Check sheet for the modelled part. Datum: model origin and axes. Units: mm. Face numbers are marked on the shaded views. A direction names the side the tool comes from. Round coordinates to 2 decimals unless told otherwise and drop trailing zeros. Order: outer loops, then holes, each group sorted by start corner. A loop starts at its lowest first (then second) coordinate and runs counter-clockwise, first axis right, second up.
(1) Thickness scan on probe 1 along X at (y, z) = (-25.5, 10); probe 2 along Y at (x, z) = (0, 3.75); probe 3 along X at (y, z) = (-20, 9.75). Record the ranges inside material, lowest first.
(2) Sectioned sample at D-D, the plane x = 42.9. Enter the section's corners in (y, z), and give its area (3 significant figures).
(3) Depth check by flat-ended pin: pin 1 (5 mm diameter, centred on x = 39, z = 5.5, fed in from +Y); pin 2 (5 mm diameter, centred on y = 0.5, z = 2, fed in from -X); pin 3 (5 mm diameter, centred on y = 19, z = 13.5, fed in from -X). Enter the tip coordinate at first touch or a pass-through.
(4) Sectioned sample at B-B, the plane y = -19. Enter the section's corners in (x, z), and give its area (3 significant figures).
(5) Tool access check on the marked faces 1, 2, 3 and 4. Record the directions out of +Z, -Z, +X, -X, +Y, -Y that give a thin tool (end or side, any length) a straight path to the whole face; none if there is none.
(6) Sectioned sample at C-C, the plane z = 5.5. Enter the section's corners in (x, y).
(7) Mould release check, pull along Y, two halves, no side actions. Record for the marked faces 5, 6 and 7: released by +Y, released by -Y, zero draft, split by the parting line, or undercut.
(8) Sectioned sample at A-A, the plane x = -12. Enter the section's corners in (y, z).
```python
from build123d import *
from build123d.topology import SkipClean

# Parameters (mm, degrees)
SKETCH1_W           = 50
SKETCH1_H           = 60
BOSS_EXTRUDE1_DEPTH = 12
SKETCH2_W           = 41
SKETCH2_H           = 4.2
CUT_EXTRUDE1_DEPTH  = 67.098411479
SKETCH3_W           = 12
SKETCH3_H           = 30
BOSS_EXTRUDE2_DEPTH = 42
SKETCH4_W           = 7.2
SKETCH4_H           = 20
CUT_EXTRUDE2_DEPTH  = 42.5
SKETCH5_R           = 2.45
CUT_EXTRUDE3_DEPTH  = 17.5
FILLET1_R           = 5
SKETCH6_R           = 2.45
CUT_EXTRUDE4_DEPTH  = 35
BOSS_EXTRUDE3_START = 5
SKETCH7_R           = 2.45
BOSS_EXTRUDE3_DEPTH = 5


with BuildPart() as part:
    # Sketch1 → Boss-Extrude1 (new body)
    with BuildSketch(Plane.XY):
        Rectangle(SKETCH1_W, SKETCH1_H)
    extrude(amount=BOSS_EXTRUDE1_DEPTH)

    # Sketch2 → Cut-Extrude1 (cut, through all)
    with BuildSketch(Plane(origin=(0, 30, 0), x_dir=(1, 0, 0), z_dir=(0, 1, 0))):
        with Locations((0, -8.9)):
            Rectangle(SKETCH2_W, SKETCH2_H)
    extrude(amount=-CUT_EXTRUDE1_DEPTH, mode=Mode.SUBTRACT)

    # Sketch3 → Boss-Extrude2 (add)
    with BuildSketch(Plane.ZY.offset(25)):
        with Locations((6, -15)):
            Rectangle(SKETCH3_W, SKETCH3_H)
    boss_extrude2 = extrude(amount=BOSS_EXTRUDE2_DEPTH)

    # Sketch4 → Cut-Extrude2 (cut)
    with BuildSketch(Plane.ZY.offset(67)):
        with Locations((7.4, -15)):
            Rectangle(SKETCH4_W, SKETCH4_H)
    cut_extrude2 = extrude(amount=-CUT_EXTRUDE2_DEPTH, mode=Mode.SUBTRACT)

    # Sketch5 → Cut-Extrude3 (cut, symmetric)
    with BuildSketch(Plane.XY.offset(12)):
        with Locations((-59.5, -14.995756269)):
            Circle(SKETCH5_R)
        with Locations((-51.2, -14.995756269)):
            Circle(SKETCH5_R)
        with Locations((-42.9, -14.995756269)):
            Circle(SKETCH5_R)
        with Locations((-34.6, -14.995756269)):
            Circle(SKETCH5_R)
    cut_extrude3 = extrude(amount=CUT_EXTRUDE3_DEPTH, both=True, mode=Mode.SUBTRACT)

    # Mirror1: Boss-Extrude2, Cut-Extrude2, Cut-Extrude3 across plane
    add(boss_extrude2.mirror(Plane(origin=(0, 0, 0), x_dir=(0, 0, 1), z_dir=(1, 0, 0))))
    add(cut_extrude2.mirror(Plane(origin=(0, 0, 0), x_dir=(0, 0, 1), z_dir=(1, 0, 0))), mode=Mode.SUBTRACT)
    add(cut_extrude3.mirror(Plane(origin=(0, 0, 0), x_dir=(0, 0, 1), z_dir=(1, 0, 0))), mode=Mode.SUBTRACT)

    # Fillet1
    # the kernel refuses this fillet: 5 mm, written as the material it adds along each edge
    with BuildSketch(Plane(origin=(25, 0, 12), x_dir=(0, 1, 0), z_dir=(0, 0, -1))) as fillet1_piece_1:
        with BuildLine():
            CenterArc((FILLET1_R, FILLET1_R), FILLET1_R, 180, 90)
            Line((0, FILLET1_R), (0, 0))
            Line((0, 0), (FILLET1_R, 0))
        make_face()
    extrude(amount=12)
    with BuildSketch(Plane(origin=(-25, 0, 12), x_dir=(0, 1, 0), z_dir=(0, 0, -1))) as fillet1_piece_2:
        with BuildLine():
            CenterArc((FILLET1_R, -FILLET1_R), FILLET1_R, 90, 90)
            Line((0, -FILLET1_R), (0, 0))
            Line((0, 0), (FILLET1_R, 0))
        make_face()
    extrude(amount=12)
    # the kernel refuses this fillet: 5 mm, written as the material it takes off along each edge
    with BuildSketch(Plane(origin=(67, 0, 24.5), x_dir=(-1, 0, 0), z_dir=(0, 0, -1)), Plane(origin=(-67, -30, -12.5), x_dir=(0, 1, 0), z_dir=(0, 0, 1)), Plane(origin=(-25, 30, -12.5), x_dir=(1, 0, 0), z_dir=(0, 0, 1))) as fillet1_2_piece_1:
        with BuildLine():
            CenterArc((FILLET1_R, -FILLET1_R), FILLET1_R, 90, 90)
            Line((0, -FILLET1_R), (0, 0))
            Line((0, 0), (FILLET1_R, 0))
        make_face()
    extrude(amount=37, mode=Mode.SUBTRACT)
    with BuildSketch(Plane(origin=(67, -30, -12.5), x_dir=(0, 1, 0), z_dir=(0, 0, 1)), Plane(origin=(-67, 0, 24.5), x_dir=(1, 0, 0), z_dir=(0, 0, -1)), Plane(origin=(25, 30, -12.5), x_dir=(-1, 0, 0), z_dir=(0, 0, 1))) as fillet1_2_piece_2:
        with BuildLine():
            CenterArc((FILLET1_R, FILLET1_R), FILLET1_R, 180, 90)
            Line((0, FILLET1_R), (0, 0))
            Line((0, 0), (FILLET1_R, 0))
        make_face()
    extrude(amount=37, mode=Mode.SUBTRACT)

    # Sketch6 → Cut-Extrude4 (cut)
    with BuildSketch(Plane.XY.offset(12)):
        Circle(SKETCH6_R)
        with Locations((0, 10)):
            Circle(SKETCH6_R)
    extrude(amount=-CUT_EXTRUDE4_DEPTH, mode=Mode.SUBTRACT)

    # Sketch7 → Boss-Extrude3 (add)
    with SkipClean():  # the faces are left unmerged after this step: merging them gives an invalid solid
        with BuildSketch(Plane.XY.offset(12).offset(BOSS_EXTRUDE3_START)):
            with BuildLine():
                ThreePointArc((-67, -25), (-65.535533906, -28.535533906), (-62, -30))
                Line((-62, -30), (62, -30))
                ThreePointArc((62, -30), (65.535533906, -28.535533906), (67, -25))
                Line((67, -25), (67, -5))
                ThreePointArc((67, -5), (65.535533906, -1.464466094), (62, 0))
                Line((62, 0), (30, 0))
                ThreePointArc((30, 0), (26.464466094, 1.464466094), (25, 5))
                Line((25, 5), (25, 25))
                ThreePointArc((25, 25), (23.535533906, 28.535533906), (20, 30))
                Line((20, 30), (-20, 30))
                ThreePointArc((-20, 30), (-23.535533906, 28.535533906), (-25, 25))
                Line((-25, 25), (-25, 5))
                ThreePointArc((-25, 5), (-26.464466094, 1.464466094), (-30, 0))
                Line((-30, 0), (-62, 0))
                ThreePointArc((-62, 0), (-65.535533906, -1.464466094), (-67, -5))
                Line((-67, -5), (-67, -25))
            make_face()
            with Locations((-59.5, -14.995756269)):
                Circle(SKETCH7_R, mode=Mode.SUBTRACT)
            with Locations((-51.2, -14.995756269)):
                Circle(SKETCH7_R, mode=Mode.SUBTRACT)
            with Locations((-42.9, -14.995756269)):
                Circle(SKETCH7_R, mode=Mode.SUBTRACT)
            with Locations((-34.6, -14.995756269)):
                Circle(SKETCH7_R, mode=Mode.SUBTRACT)
            with Locations((59.5, -14.995756269)):
                Circle(SKETCH7_R, mode=Mode.SUBTRACT)
            with Locations((51.2, -14.995756269)):
                Circle(SKETCH7_R, mode=Mode.SUBTRACT)
            with Locations((42.9, -14.995756269)):
                Circle(SKETCH7_R, mode=Mode.SUBTRACT)
            with Locations((34.6, -14.995756269)):
                Circle(SKETCH7_R, mode=Mode.SUBTRACT)
            with Locations((0, 10)):
                Circle(SKETCH7_R, mode=Mode.SUBTRACT)
            Circle(SKETCH7_R, mode=Mode.SUBTRACT)
        extrude(amount=-BOSS_EXTRUDE3_DEPTH)


solid = part.part
```
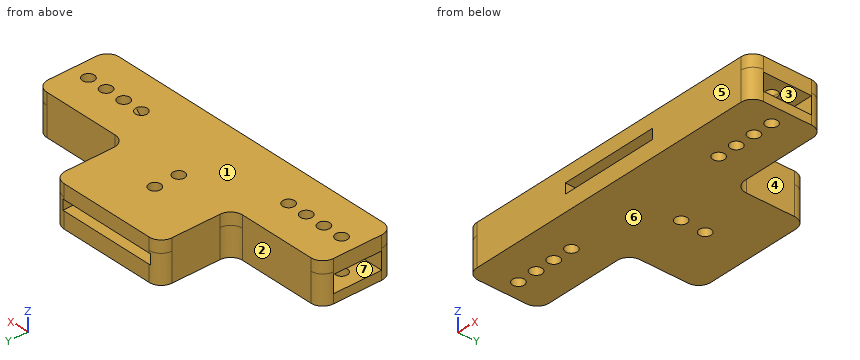
Derived:
1. probe 1: x = -66.97 to -20.5, 20.5 to 66.97
1. probe 2: y = -30 to -2.45, 2.45 to 7.55, 12.45 to 30
1. probe 3: x = -24.5 to -20.5, 20.5 to 24.5
2. outline: (-30, 0) - (-17.45, 0) - (-17.45, 3.8) - (-25, 3.8) - (-25, 11) - (-17.45, 11) - (-17.45, 17) - (-30, 17) - close; (-12.55, 0) - (0, 0) - (0, 17) - (-12.55, 17) - (-12.55, 11) - (-5, 11) - (-5, 3.8) - (-12.55, 3.8) - close
2. area: 318 mm2
3. pin 1: stops at y = 0
3. pin 2: stops at x = -66
3. pin 3: stops at x = -25
4. outline: (-67, 0) - (67, 0) - (67, 3.8) - (24.5, 3.8) - (24.5, 11) - (67, 11) - (67, 17) - (-67, 17) - (-67, 11) - (-24.5, 11) - (-24.5, 3.8) - (-67, 3.8) - close; hole (-20.5, 6.8) - (20.5, 6.8) - (20.5, 11) - (-20.5, 11) - close
4. area: 1,490 mm2
5. face 1: +Z, +X, -X, +Y, -Y
5. face 2: +Z, -Z, -X, +Y
5. face 3: +X
5. face 4: +Z, -Z, +X, +Y
6. outline: (-67, -25) arc R5 ccw to (-62, -30) - (62, -30) arc R5 ccw to (67, -25) - (24.5, -25) - (24.5, -5) - (67, -5) arc R5 ccw to (62, 0) - (30, 0) arc R5 cw to (25, 5) - (25, 25) arc R5 ccw to (20, 30) - (-20, 30) arc R5 ccw to (-25, 25) - (-25, 5) arc R5 cw to (-30, 0) - (-62, 0) arc R5 ccw to (-67, -5) - (-24.5, -5) - (-24.5, -25) - close; hole circle Ø4.9 at (0, 0); hole circle Ø4.9 at (0, 10)
7. face 5: released by -Y
7. face 6: zero draft
7. face 7: undercut
8. outline: (-30, 0) - (30, 0) - (30, 6.8) - (-30, 6.8) - close; (-30, 11) - (30, 11) - (30, 17) - (-30, 17) - close
